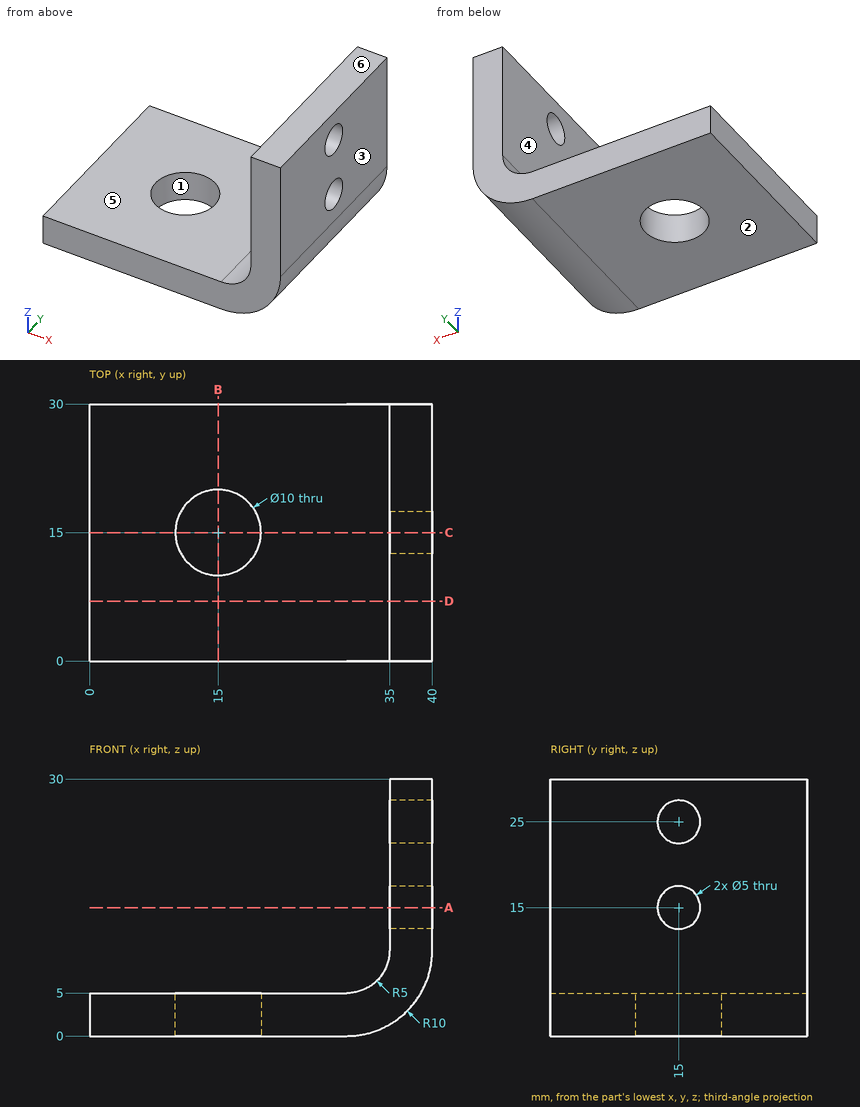
Here's the drawing with two shaded views (mm, measured from the low corner). I have some questions. A direction names the side the tool comes from. Coordinates: 2 decimals unless noted, no trailing zeros. Loops run counter-clockwise (first coordinate to the right, second up) from the corner with the lowest first, then second, coordinate; pieces in that order, holes last. Notation, with made-up numbers: M 86.5,-20.75 L 121.5,-20.75 A5 cw 121.5,-14.75 Z; hole C 30,-36 d4. An arc over 180 degrees is marked long. Answer as CSV lines item,"result". Start each with the question number.
1. Suppose I cut it at D-D, the plane y = 7. List the corners of the cut face in (x, z) for me, plus the area to 3 significant figures.
2. For pin 1 Ø4.5 at (y, z) = (15, 25) entering from -X; pin 2 Ø1 at (x, y) = (7.5, 11) entering from +Z; pin 3 Ø8 at (y, z) = (26, 4.5) entering from +X; pin 4 Ø6 at (y, z) = (4, 3.5) entering from +X, each with a flat end and sliding along its axis, tell me the tip position at first contact or that it passes through.
3. Suppose I cut it at A-A, the plane z = 15. List the corners of the cut face in (x, y) for me.
4. If I drill on probe 1 along Z at (x, y) = (37.35, 15); probe 2 along Z at (x, y) = (38.7, 15); probe 3 along Y at (x, z) = (15, 1.65), over which ranges is the centre line in solid material (lowest first)? Write a range as [from, to].
5. Thinking about a two-plate mould opening in X: for the marked faces 1, 2, 3 and 4, which applies, +X half, -X half, draft (parallel to the pull), parting line (faces both ways), or undercut?
6. Suppose I cut it at C-C, the plane y = 15. List the corners of the cut face in (x, z) for me, plus the area to 3 significant figures.
7. Suppose I cut it at B-B, the plane x = 15. List the corners of the cut face in (y, z) for me.
8. For the marked faces 5 and 6, which set-ups out of +Z, -Z, +X, -X, +Y, -Y let a thin tool reach every point of the face, with its end or its side?
Output:
1,outline,"M 0,0 L 30,0 A10 ccw 40,10 L 40,30 L 35,30 L 35,10 A5 cw 30,5 L 0,5 Z"
1,area,"309 mm^2"
2,pin 1,"passes through"
2,pin 2,"stops at z = 5"
2,pin 3,"stops at x = 39.89"
2,pin 4,"stops at x = 39.37"
3,outline,"M 35,0 L 40,0 L 40,12.5 L 35,12.5 Z; M 35,17.5 L 40,17.5 L 40,30 L 35,30 Z"
4,probe 1,"z = [3.22, 12.5], [17.5, 22.5], [27.5, 30]"
4,probe 2,"z = [5.07, 12.5], [17.5, 22.5], [27.5, 30]"
4,probe 3,"y = [0, 10], [20, 30]"
5,face 1,"undercut"
5,face 2,"draft"
5,face 3,"+X half"
5,face 4,"-X half"
6,outline,"M 0,0 L 10,0 L 10,5 L 0,5 Z; M 20,0 L 30,0 A10 ccw 40,10 L 40,12.5 L 35,12.5 L 35,10 A5 cw 30,5 L 20,5 Z; M 35,17.5 L 40,17.5 L 40,22.5 L 35,22.5 Z; M 35,27.5 L 40,27.5 L 40,30 L 35,30 Z"
6,area,"209 mm^2"
7,outline,"M 0,0 L 10,0 L 10,5 L 0,5 Z; M 20,0 L 30,0 L 30,5 L 20,5 Z"
8,face 5,"+Z, -X, +Y, -Y"
8,face 6,"+Z, +X, -X, +Y, -Y"
